Autodesk Inventor part; units mm, degrees
ref_plane "YZ Plane" through (0, 0, 0) normal (1, 0, 0) x (0, 1, 0)
ref_plane "XZ Plane" through (0, 0, 0) normal (0, 1, 0) x (-1, 0, 0)
ref_plane "XY Plane" through (0, 0, 0) normal (0, 0, 1) x (1, 0, 0)
sketch "草图1" plane through (0, 0, 0) normal (0, 1, 0) x (-1, 0, 0)
  line L0 (3, -60) -> (0, -60)
  line L1 (0, -60) -> (0, 0)
  line L2 (45.4264, -42.4264) -> (47.5477, -40.3051)
  line L3 (47.5477, -40.3051) -> (0, 7.2426)
  line L4 (0, 0) -> (0, 7.2426)
  line L5 (3, -22.3594) -> (18.8105, -15.8105)
  line L6 (21.1066, -18.1066) -> (3, -25.6066)
  line L7 (3, 0) -> (18.8105, -15.8105)
  line L8 (21.1066, -18.1066) -> (45.4264, -42.4264)
  line L9 (3, 0) -> (3, -22.3594)
  line L10 (3, -25.6066) -> (3, -60)
  dimension "d3" = 60
  dimension "d6" = 3
extrude "拉伸1" add sketch "草图1" along normal blind 42
sketch "草图2" plane through (-47.5477, 0, -40.3051) normal (-0.7071, 0, -0.7071) x (-0.7071, 0, 0.7071)
  line L0 (-3, 0) -> (0, 0)
  line L1 (0, 0) -> (0, 42)
  line L2 (-3, 42) -> (0, 42)
  line L3 (-3, 0) -> (-3, 42)
  point P0 (-5.1213, 0)
extrude "拉伸2" add sketch "草图2" along normal blind 42
sketch "草图3" plane through (-21.1066, 0, -18.1066) normal (0.7071, 0, -0.7071) x (-0.7071, 0, -0.7071)
  line L0 (0, 0) -> (76.3934, 0)
  line L1 (76.3934, 42) -> (76.3934, 0)
  line L2 (0, 42) -> (76.3934, 42)
  line L3 (0, 0) -> (0, 42)
  circle A0 centre (55.3934, 21) radius 15
  point P0 (-27.7279, 0)
  dimension "d11" = 30
  dimension "d12" = 21
  dimension "d13" = 21
extrude "拉伸3" cut sketch "草图3" against normal blind 42 contours A0
properties part number "45度角件" material "钢"
For this review, take the finished solid that the model builds, in its own axes (mm). A direction names the side the tool comes from. Give positions to 0.01 mm unless a question says otherwise; leave off trailing zeros. Write each loop counter-clockwise with the first axis right and the second up, starting at its lowest first coordinate (ties: lowest second). Pieces come first, ordered by that corner, then holes. Notation, with made-up numbers: M 23,22.5 L 52,22.5 A11 cw 52,43.5 Z; hole C 0,68 d8. An arc over 180 degrees is marked long. Answer as a JSON object with one key per item and string values. Group by question number.
Item 1: Consider section B-B on x = -12. Write out the cut boundary in (y, z).
Item 2: For probe 1 along X at (y, z) = (29, -52.5); probe 2 along X at (y, z) = (30, -2.5); probe 3 along Z at (x, y) = (-12.5, 36), list the stretches that pass through material, from the lowest coordinate up. Write a range as [from, to].
Item 3: Consider section A-A on y = 8.5. Count the separate pieces of the cut face and the enclosed holes in it, plus the area to 3 significant figures.
Item 4: For pin 1 Ø4 at (x, y) = (-53, 25.5) entering from +Z; pin 2 Ø10 at (x, y) = (-14, 12) entering from -Z; pin 3 Ø10 at (x, y) = (-49, 9.5) entering from -Z, all flat-tipped, find the tip position at first contact; note any pin that passes through.
Item 5: Tool access review of faces 4 (the flat face through (-27, 0, -23)), 5 (the flat face through (-50, 16, -47)), 6 (the flat face through (-3, 21, -11)), 7 (the flat face through (-2, 21, -60)): name each direction out of +Z, -Z, +X, -X, +Y, -Y from which nothing blocks a thin tool from reaching the whole face with its end or side.
Item 6: Consider section C-C on z = -17. Write out the cut boundary in (x, y).
Item 7: Draft analysis for pull direction X (two halves, no side actions). For faces 1 (the flat face through (-11, 21, -8)), 2 (the flat face through (-39.16, 20.71, -31.92)), 3 (the flat face through (-27, 42, -23)), state which applies: +X half, -X half, draft (parallel to the pull), parting line (faces both ways), or undercut.
Check result:
{
 "1": {"outline": "M 0,-21.88 L 42,-21.88 L 42,-18.63 L 0,-18.63 Z; M 0,-9 L 42,-9 L 42,-4.76 L 0,-4.76 Z"},
 "2": {"probe 1": "x = [-3, 0]", "probe 2": "x = [-9.74, -5.5], [-3, 0]", "probe 3": "z = [-21.67, -18.42], [-9.5, -5.26]"},
 "3": {"separate pieces": "2", "enclosed holes": "1", "area": "513 mm^2"},
 "4": {"pin 1": "stops at z = -43.76", "pin 2": "stops at z = -23.12", "pin 3": "stops at z = -50.97"},
 "5": {"face 4": "+Z, -Z, +X, -X, -Y", "face 5": "-Z, +Y, -Y", "face 6": "+Y, -Y", "face 7": "-Z, +X, +Y, -Y"},
 "6": {"outline": "M -24.24,0 L -15.94,0 L -15.94,42 L -24.24,42 Z; M -3,0 L 0,0 L 0,42 L -3,42 Z"},
 "7": {"face 1": "undercut", "face 2": "-X half", "face 3": "draft"}
}
